Autodesk Inventor part; units mm, degrees
ref_plane "YZ Plane" through (0, 0, 0) normal (1, 0, 0) x (0, 1, 0)
ref_plane "XZ Plane" through (0, 0, 0) normal (0, 1, 0) x (-1, 0, 0)
ref_plane "XY Plane" through (0, 0, 0) normal (0, 0, 1) x (1, 0, 0)
sketch "Sketch1" plane through (0, 0, 0) normal (0, 1, 0) x (-1, 0, 0)
  line L0 (0, 0) -> (25.4, 0)
  line L1 (25.4, 0) -> (25.4, 25.4)
  line L2 (25.4, 25.4) -> (0, 25.4)
  line L3 (0, 25.4) -> (0, 0)
  line L4 (1.651, 1.651) -> (23.749, 1.651)
  line L5 (23.749, 1.651) -> (23.749, 23.749)
  line L6 (23.749, 23.749) -> (1.651, 23.749)
  line L7 (1.651, 23.749) -> (1.651, 1.651)
  dimension "d0" = 25.4
  dimension "d1" = 25.4
  dimension "d2" = 1.651
  dimension "d3" = 1.651
  dimension "d4" = 1.651
  dimension "d5" = 1.651
extrude "Extrusion1" add sketch "Sketch1" along normal blind 317.5
sketch "Sketch3" plane through (-25.4, 0, 25.4) normal (0, 0, 1) x (1, 0, 0)
  line L0 (0, 0) -> (25.4, 0)
  line L1 (25.4, 0) -> (25.4, 317.5)
  line L2 (0, 317.5) -> (25.4, 317.5)
  line L3 (0, 0) -> (0, 317.5)
sketch "Sketch4" plane through (-25.4, 0, 25.4) normal (0, 0, 1) x (1, 0, 0)
  line L0 (0, 0) -> (25.4, 0)
  line L1 (25.4, 0) -> (25.4, 317.5)
  point P0 (12.7, 12.7)
  point P1 (12.7, 63.5)
  dimension "d12" = 12.7
  dimension "d13" = 12.7
  dimension "d14" = 12.7
  dimension "d15" = 50.8
hole "Hole1" at (-12.7, 12.7, 25.4) direction (0, 0, -1) diameter 6.35 end through all
sketch "Sketch5" plane through (-25.4, 0, 25.4) normal (0, 0, 1) x (1, 0, 0)
  circle A0 centre (12.7, 12.7) radius 3.175
  line L0 (25.4, 0) -> (25.4, 317.5)
  point P0 (12.7, 63.5)
  dimension "d23" = 12.7
  dimension "d24" = 50.8
hole "Hole2" at (-12.7, 63.5, 25.4) direction (0, 0, -1) diameter 6.35 end through all
sketch "Sketch6" plane through (0, 0, 25.4) normal (1, 0, 0) x (0, 0, -1)
  line L0 (0, 0) -> (25.4, 0)
  line L1 (25.4, 0) -> (25.4, 317.5)
  point P0 (12.7, 19.05)
  point P1 (12.7, 44.45)
  dimension "d32" = 12.7
  dimension "d33" = 12.7
  dimension "d34" = 19.05
  dimension "d35" = 25.4
hole "Hole3" at (0, 19.05, 12.7) at (0, 44.45, 12.7) direction (-1, 0, 0) diameter 6.35 end through all
sketch "Sketch7" plane through (0, 0, 25.4) normal (1, 0, 0) x (0, 0, -1)
  line L0 (0, 317.5) -> (25.4, 317.5)
  line L1 (0, 0) -> (0, 317.5)
  point P0 (12.7, 304.8)
  dimension "d43" = 12.7
  dimension "d44" = 12.7
hole "Hole4" at (0, 304.8, 12.7) direction (-1, 0, 0) diameter 9.525 end through all
properties part number "Front_Bar" material "Aluminum 6061"
Verification items for the finished model (mm, model axes). A direction names the side the tool comes from. Round coordinates to 2 decimals unless told otherwise and drop trailing zeros. Write each loop counter-clockwise with the first axis right and the second up, starting at its lowest first coordinate (ties: lowest second). Pieces come first, ordered by that corner, then holes. Notation, with made-up numbers: (70, 46.5) - (127, 46.5) arc R17 ccw to (127, 61.5) - close; hole circle Ø8 at (72, -10.75). An arc over 180 degrees is marked (long way). Answer as a JSON object with one key per item and string values. Group by question number.
Q1. Thickness scan on line 1 (Z direction, x = -24.4, y = 44.45) (3 decimals); line 2 (X direction, y = 286, z = 10.75); line 3 (Z direction, x = -10.25, y = 265.5). Record the ranges inside material, lowest first.
Q2. Section check A-A, the plane z = 21. Enter the section's corners in (x, y), plus the area to 3 significant figures.
Q3. Mould release check, pull along Z, two halves, no side actions. Record for faces 3 (the cylindrical face through (-0.84, 309.45, 13.73)), 4 (the flat face through (-13, 157, 0)), 5 (the flat face through (0, 157, 13)): released by +Z, released by -Z, zero draft, split by the parting line, or undercut.
Q4. Section check B-B, the plane y = 275. Enter the section's corners in (x, z), plus the area to 3 significant figures.
Q5. Section check D-D, the plane y = 63.5. Enter the section's corners in (x, z) (3 decimals), plus the area to 3 significant figures.
Q6. Section check C-C, the plane x = -12.7. Enter the section's corners in (y, z) (3 decimals), plus the area to 3 significant figures.
Q7. Tool access check on faces 1 (the cylindrical face through (-11.48, 60.57, 24.56)), 2 (the flat face through (-13, 157, 23.749)). Record the directions out of +Z, -Z, +X, -X, +Y, -Y that give a thin tool (end or side, any length) a straight path to the whole face; none if there is none.
Found:
{
 "1": {"line 1": "z = 0 to 9.525, 15.875 to 25.4", "line 2": "x = -25.4 to -23.75, -1.65 to 0", "line 3": "z = 0 to 1.65, 23.75 to 25.4"},
 "2": {"outline": "(-25.4, 0) - (-23.75, 0) - (-23.75, 317.5) - (-25.4, 317.5) - close; (-1.65, 0) - (0, 0) - (0, 317.5) - (-1.65, 317.5) - close", "area": "1,050 mm^2"},
 "3": {"face 3": "undercut", "face 4": "released by -Z", "face 5": "zero draft"},
 "4": {"outline": "(-25.4, 0) - (0, 0) - (0, 25.4) - (-25.4, 25.4) - close; hole (-23.75, 1.65) - (-1.65, 1.65) - (-1.65, 23.75) - (-23.75, 23.75) - close", "area": "157 mm^2"},
 "5": {"outline": "(-25.4, 0) - (-15.875, 0) - (-15.875, 1.651) - (-23.749, 1.651) - (-23.749, 23.749) - (-15.875, 23.749) - (-15.875, 25.4) - (-25.4, 25.4) - close; (-9.525, 0) - (0, 0) - (0, 25.4) - (-9.525, 25.4) - (-9.525, 23.749) - (-1.651, 23.749) - (-1.651, 1.651) - (-9.525, 1.651) - close", "area": "136 mm^2"},
 "6": {"outline": "(0, 0) - (9.525, 0) - (9.525, 1.651) - (0, 1.651) - close; (0, 23.749) - (9.525, 23.749) - (9.525, 25.4) - (0, 25.4) - close; (15.875, 0) - (60.325, 0) - (60.325, 1.651) - (15.875, 1.651) - close; (15.875, 23.749) - (60.325, 23.749) - (60.325, 25.4) - (15.875, 25.4) - close; (66.675, 0) - (317.5, 0) - (317.5, 1.651) - (66.675, 1.651) - close; (66.675, 23.749) - (317.5, 23.749) - (317.5, 25.4) - (66.675, 25.4) - close", "area": "1,010 mm^2"},
 "7": {"face 1": "+Z, -Z", "face 2": "+Y, -Y"}
}
